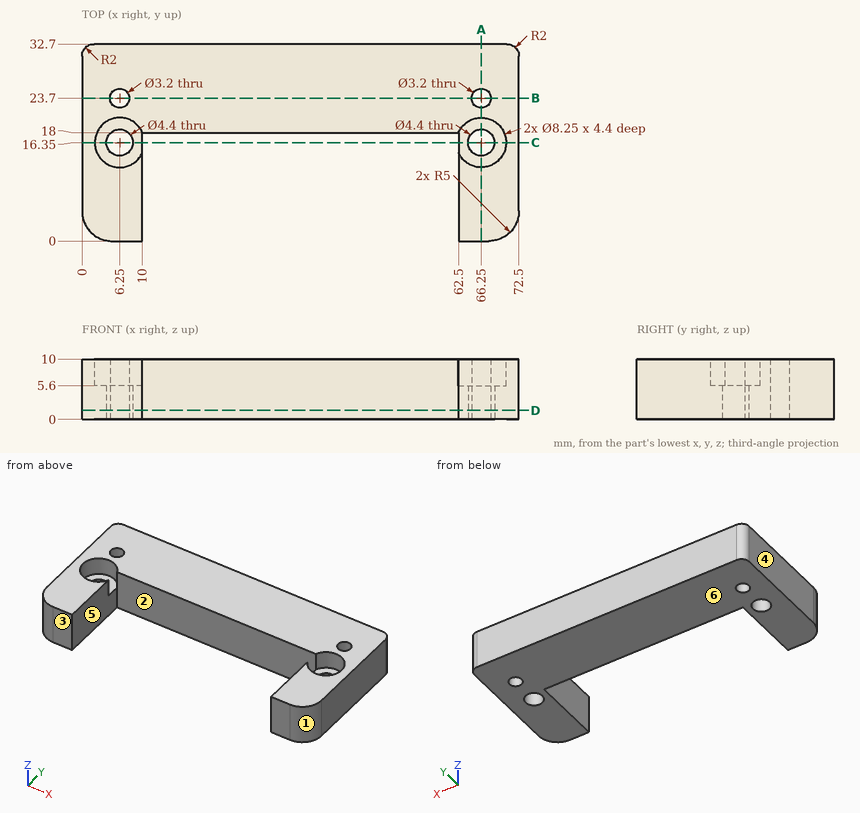
Check sheet for the drawn part. Datum: minimum x, y, z corner. Units: mm. A direction names the side the tool comes from. Coordinates: 2 decimals unless noted, no trailing zeros. Write each loop counter-clockwise with the first axis right and the second up, starting at its lowest first coordinate (ties: lowest second). Pieces come first, ordered by that corner, then holes. Notation, with made-up numbers: (86, -1.75) - (128, -1.75) arc R18 ccw to (128, 8.25) - close; hole circle Ø2 at (43, 75.25). An arc over 180 degrees is marked (long way). Answer as a JSON object with one key per item and string values.
(1) Mould release check, pull along X, two halves, no side actions. Record for the marked faces 1, 2, 3 and 4: pulls with the +X half, pulls with the -X half, needs draft (parallel to the pull), parting line crosses it, or undercut.
Report:
{"face 1": "pulls with the +X half", "face 2": "undercut", "face 3": "needs draft", "face 4": "pulls with the -X half"}
(2) Cross-section at C-C on y = 16.35. Record the cut outline in (x, z) (3 decimals).
Report:
{"outline": "(0, 0) - (4.05, 0) - (4.05, 5.6) - (2.125, 5.6) - (2.125, 10) - (0, 10) - close; (8.45, 0) - (10, 0) - (10, 5.6) - (8.45, 5.6) - close; (62.5, 0) - (64.05, 0) - (64.05, 5.6) - (62.5, 5.6) - close; (68.45, 0) - (72.5, 0) - (72.5, 10) - (70.375, 10) - (70.375, 5.6) - (68.45, 5.6) - close"}
(3) Cross-section at D-D on z = 1.5. Record the cut outline in (x, y).
Report:
{"outline": "(0, 5) arc R5 ccw to (5, 0) - (10, 0) - (10, 18) - (62.5, 18) - (62.5, 0) - (67.5, 0) arc R5 ccw to (72.5, 5) - (72.5, 30.7) arc R2 ccw to (70.5, 32.7) - (2, 32.7) arc R2 ccw to (0, 30.7) - close; hole circle Ø4.4 at (6.25, 16.35); hole circle Ø3.2 at (6.25, 23.7); hole circle Ø4.4 at (66.25, 16.35); hole circle Ø3.2 at (66.25, 23.7)"}
(4) Thickness scan on line 1 along Y through (x, z) = (66.25, 6.8) (3 decimals); line 2 along Y through (x, z) = (6.25, 3.25); line 3 along X through (y, z) = (25, 5.25). Record the ranges inside material, lowest first.
Report:
{"line 1": "0 to 12.225, 20.475 to 22.1, 25.3 to 32.7", "line 2": "0 to 14.15, 18.55 to 22.1, 25.3 to 32.7", "line 3": "0 to 5.32, 7.18 to 65.32, 67.18 to 72.5"}
(5) Cross-section at B-B on y = 23.7. Record the cut outline in (x, z).
Report:
{"outline": "(0, 0) - (4.65, 0) - (4.65, 10) - (0, 10) - close; (7.85, 0) - (64.65, 0) - (64.65, 10) - (7.85, 10) - close; (67.85, 0) - (72.5, 0) - (72.5, 10) - (67.85, 10) - close"}
(6) Cross-section at A-A on x = 66.25. Record the cut outline in (y, z) (3 decimals).
Report:
{"outline": "(0, 0) - (14.15, 0) - (14.15, 5.6) - (12.225, 5.6) - (12.225, 10) - (0, 10) - close; (18.55, 0) - (22.1, 0) - (22.1, 10) - (20.475, 10) - (20.475, 5.6) - (18.55, 5.6) - close; (25.3, 0) - (32.7, 0) - (32.7, 10) - (25.3, 10) - close"}
(7) Tool access check on the marked faces 5 and 6. Record the directions out of +Z, -Z, +X, -X, +Y, -Y that give a thin tool (end or side, any length) a straight path to the whole face; none if there is none.
Report:
{"face 5": "+Z, -Z, -Y", "face 6": "-Z, +X, -X, +Y, -Y"}
(8) Gauge pin test, flat ends, axial feed: pin 1 Ø2.5 at (x, y) = (4.5, 14.5) entering from +Z; pin 2 Ø1 at (x, z) = (47.5, 8) entering from -Y; pin 3 Ø3 at (x, y) = (6.25, 23.7) entering from -Z. Record the tip position at first contact, or that the pin passes through.
Report:
{"pin 1": "z = 5.6", "pin 2": "y = 18", "pin 3": "through"}
